from build123d import *

# Parameters (mm, degrees)
F1_DEPTH = 15
F3_DEPTH = 28.0871216252
F4_R     = 2
F5_DEPTH = 5
F6_R     = 4
F7_DEPTH = 54.001


with BuildPart() as f1:
    # F0 (on Front) → F1 (new body, symmetric)
    with BuildSketch(Plane.XZ):
        with BuildLine():
            Line((-25, 25), (-25, 0))
            ThreePointArc((-25, 0), (0, -25), (25, 0))
            Line((25, 0), (25, 25))
            Line((25, 25), (20, 25))
            Line((20, 25), (20, 0))
            ThreePointArc((20, 0), (0, -20), (-20, 0))
            Line((-20, 0), (-20, 25))
            Line((-20, 25), (-25, 25))
        make_face()
    extrude(amount=F1_DEPTH, both=True)



with BuildPart() as f1b:
    # F0 (on Front) → F1, piece 2 (new body, symmetric)
    with BuildSketch(Plane.XZ):
        with BuildLine():
            Line((14, -50), (0, -50))
            Line((0, -50), (-14, -50))
            ThreePointArc((-14, -50), (-15.4142135624, -49.4142135624), (-16, -48))
            Line((-16, -48), (-16, -43))
            ThreePointArc((-16, -43), (-17.4644660941, -39.4644660941), (-21, -38))
            Line((-21, -38), (-29, -38))
            Line((-29, -38), (-29, -43))
            Line((-29, -43), (-23, -43))
            ThreePointArc((-23, -43), (-21.5857864376, -43.5857864376), (-21, -45))
            Line((-21, -45), (-21, -48))
            ThreePointArc((-21, -48), (-18.9497474683, -52.9497474683), (-14, -55))
            Line((-14, -55), (14, -55))
            ThreePointArc((14, -55), (18.9497474683, -52.9497474683), (21, -48))
            Line((21, -48), (21, -45))
            ThreePointArc((21, -45), (21.5857864376, -43.5857864376), (23, -43))
            Line((23, -43), (29, -43))
            Line((29, -43), (29, -38))
            Line((29, -38), (21, -38))
            ThreePointArc((21, -38), (17.4644660941, -39.4644660941), (16, -43))
            Line((16, -43), (16, -48))
            ThreePointArc((16, -48), (15.4142135624, -49.4142135624), (14, -50))
        make_face()
    extrude(amount=F1_DEPTH, both=True)


with BuildPart() as f1_1:
    add(f1.part)

    add(f1b.part)  # F3 merges F1b
    # F2 (on face) → F3 (join, up to face)
    with BuildSketch(Plane.XY.offset(-50)):
        with BuildLine():
            ThreePointArc((7.5, -2.5), (10, 0), (7.5, 2.5))
            Line((7.5, 2.5), (2.5, 2.5))
            Line((2.5, 2.5), (2.5, 7.5))
            ThreePointArc((2.5, 7.5), (0, 10), (-2.5, 7.5))
            Line((-2.5, 7.5), (-2.5, 2.5))
            Line((-2.5, 2.5), (-7.5, 2.5))
            ThreePointArc((-7.5, 2.5), (-10, 0), (-7.5, -2.5))
            Line((-7.5, -2.5), (-2.5, -2.5))
            Line((-2.5, -2.5), (-2.5, -7.5))
            ThreePointArc((-2.5, -7.5), (0, -10), (2.5, -7.5))
            Line((2.5, -7.5), (2.5, -2.5))
            Line((2.5, -2.5), (7.5, -2.5))
        make_face()
    extrude(amount=F3_DEPTH)

    # F4 (on face) → F5 (cut, through all)
    with BuildSketch(Plane(origin=(0, 0, -43), x_dir=(1, 0, 0), z_dir=(0, 0, -1))):
        with Locations((-26, -10)):
            Circle(F4_R)
        with Locations((-26, 0)):
            Circle(F4_R)
        with Locations((-26, 10)):
            Circle(F4_R)
        with Locations((26, -10)):
            Circle(F4_R)
        with Locations((26, 0)):
            Circle(F4_R)
        with Locations((26, 10)):
            Circle(F4_R)
    extrude(amount=-F5_DEPTH, mode=Mode.SUBTRACT)

    # F6 (on face) → F7 (cut, through all)
    with BuildSketch(Plane.YZ.offset(25)):
        with Locations((-7, 5)):
            Circle(F6_R)
        with Locations((7, 15)):
            Circle(F6_R)
    extrude(amount=-F7_DEPTH, mode=Mode.SUBTRACT)


solid = f1_1.part
CAD build for the part. Positions are in the model's coordinates, mm. A direction names the side the tool comes from. Round coordinates to 2 decimals unless told otherwise and drop trailing zeros. Loops run counter-clockwise (first coordinate to the right, second up) from the corner with the lowest first, then second, coordinate; pieces in that order, holes last.
(1) Drop flat-ended pins along their axis: pin 1 (2.5 mm diameter, centred on y = 7, z = -46, fed in from -X); pin 2 (8 mm diameter, centred on x = 8.5, y = -1, fed in from +Z); pin 3 (5.5 mm diameter, centred on y = -7, z = -46, fed in from +X). Give the stop position or say it passes through.
(2) Wall check: line 1 along Y through (x, z) = (-26, -41.55); line 2 along X through (y, z) = (3, 21); line 3 along X through (y, z) = (0, -39.4). Give the ranges that are in metal, low to high.
(3) Cut at C-C (x = 0). Give the cut face in (y, z).
(4) Which spindle directions (+Z, -Z, +X, -X, +Y, -Y) get a long thin tool onto all of the face, cutting with end or side? Do faces 5 (the cylindrical face through (8.032, -3.543, -23.675)), 6 (the flat face through (-2.5, 5, -38)), 7 (the flat face through (23, 0, -38)), 8 (the cylindrical face through (18, 0, -39)), 9 (the flat face through (-21, 0, -46)). Say none if no direction does.
(5) Cut at B-B (x = -22). Give the cut face in (y, z).
(6) Cut at D-D (z = -7.5). Give the cut face in (x, y).
(7) Two-plate mould, pull along Y, no slides. Class faces 1 (the cylindrical face through (27.908, -0.601, -40.535)), 2 (the flat face through (-25, 0, 13)), 3 (the cylindrical face through (-26, -12, -41)), 4 (the flat face through (-5, -2.5, -37)): +Y half, -Y half, draft (parallel to the pull), parting line (faces both ways), or undercut.
(8) Cut at A-A (z = 15). Give the cut face in (x, y), plus the area to 3 significant figures.
Findings below:
1. pin 1: stops at x = -21.02
1. pin 2: stops at z = -15.61
1. pin 3: stops at x = 22.03
2. line 1: y = -15 to -12, -8 to -2, 2 to 8, 12 to 15
2. line 2: x = -25 to -20, 20 to 25
2. line 3: x = -29 to -28, -24 to -17.53, -10 to 10, 17.53 to 24, 28 to 29
3. outline: (-15, -55) - (15, -55) - (15, -50) - (10, -50) - (10, -25) - (15, -25) - (15, -20) - (-15, -20) - (-15, -25) - (-10, -25) - (-10, -50) - (-15, -50) - close
4. face 5: none
4. face 6: +Y
4. face 7: +X, +Y, -Y
4. face 8: +Y, -Y
4. face 9: -Z, -X, +Y, -Y
5. outline: (-15, -43.27) - (15, -43.27) - (15, -38) - (-15, -38) - close; (-15, -11.87) - (15, -11.87) - (15, 25) - (-15, 25) - close; hole circle Ø8 at (-7, 5); hole circle Ø8 at (7, 15)
6. outline: (-23.85, -15) - (-18.54, -15) - (-18.54, 15) - (-23.85, 15) - close; (18.54, -15) - (23.85, -15) - (23.85, 15) - (18.54, 15) - close
7. face 1: undercut
7. face 2: draft
7. face 3: undercut
7. face 4: -Y half
8. outline: (-25, -15) - (-20, -15) - (-20, 3) - (-25, 3) - close; (-25, 11) - (-20, 11) - (-20, 15) - (-25, 15) - close; (20, -15) - (25, -15) - (25, 3) - (20, 3) - close; (20, 11) - (25, 11) - (25, 15) - (20, 15) - close
8. area: 220 mm2
